For this review, take the finished solid that the model builds, in its own axes (mm). A direction names the side the tool comes from. Coordinates: 2 decimals unless noted, no trailing zeros. Order: outer loops, then holes, each group sorted by start corner. A loop starts at its lowest first (then second) coordinate and runs counter-clockwise, first axis right, second up. Notation, with made-up numbers: (67, 77) -> (93, 77) arc R20 cw to (93, 106) -> close; hole circle Ø6 at (59, 30.25). An arc over 180 degrees is marked (long way). Return JSON: item names as keys, results as strings. Group by question number.
Item 1: Take a section at B-B (z = -8.3). Write out the cut boundary in (x, y), then the cut area to 3 significant figures.
Item 2: Machinability: for faces 4 (the flat face through (11.1, 15, 2.4)), 5 (the cylindrical face through (21.2, 1.48, 11.65)), 6 (the cylindrical face through (-22, 3.04, -21.87)), 7 (the flat face through (-13.5, 11, -4)), 8 (the flat face through (0, 0, 0)), which of the approach directions +Z, -Z, +X, -X, +Y, -Y give a long, thin tool a straight path to every point of the face, cutting with its end or side? Answer none if there is none.
Item 3: For line 1 along Z through (x, y) = (18.5, 4.65); line 2 along X through (y, z) = (1.55, -17.3); line 3 along Z through (x, y) = (3, 2.35), list the stretches that pass through material, from the lowest coordinate up.
Item 4: Take a section at D-D (y = 12.5). Write out the cut boundary in (x, z).
Item 5: Draft analysis for pull direction X (two halves, no side actions). For faces 1 (the flat face through (0, 8, -23.3)), 2 (the cylindrical face through (20.696, 4.521, -16.812)), 3 (the cylindrical face through (-22, 3.04, 13.27)), state which applies: +X half, -X half, draft (parallel to the pull), parting line (faces both ways), or undercut.
Item 6: Take a section at C-C (x = 5.5). Write out the cut boundary in (y, z), then the cut area to 3 significant figures.
Item 7: Take a section at A-A (x = 0). Write out the cut boundary in (y, z).
Item 8: Insertion check: pin 1 (7.5 mm diameter, centred on x = 2.5, z = -2.5, fed in from +Y); pin 2 (3.5 mm diameter, centred on y = 12.5, z = 2, fed in from -X); pin 3 (5 mm diameter, centred on x = -18.5, z = 8.7, fed in from -Y). Each pin has a flat end and moves straight along its axis. Give the tip position at first contact, or say it passes through.
```python
from build123d import *

# Parameters (mm, degrees)
SKETCH_1_W          = 27
SKETCH_1_H          = 38
SKETCH_1_R          = 7.5
SKETCH_1_R_2        = 3.5
SKETCH_1_R_3        = 1.5
EXTRUDE_1_DEPTH     = 3
SKETCH_4_W          = 10
SKETCH_4_H          = 6
EXTRUDE_3_DEPTH     = 38
SKETCH_6_R          = 2.5
CUT_EXTRUDE_3_DEPTH = 1
EXTRUDE_4_OUTLINE_W = 27
EXTRUDE_4_OUTLINE_H = 38
EXTRUDE_4_DEPTH     = 14
SKETCH_13_R         = 2.25
CUT_EXTRUDE_6_DEPTH = 10
CUT_EXTRUDE_8_DEPTH = 2
FILLET_1_R          = 5
SKETCH_17_R         = 4
CUT_EXTRUDE_9_DEPTH = 3


# Read off the part's stored shape, not the designer's step: 凸台-拉伸4
with BuildPart() as part:
    # 草图1 → 凸台-拉伸1 (new body)
    with BuildSketch(Plane(origin=(0, 0, 0), x_dir=(1, 0, 0), z_dir=(0, 1, 0))):
        with Locations((0, 4.3)):
            Rectangle(SKETCH_1_W, SKETCH_1_H)
        with Locations(Location((0, 8.3, 0), (0, 0, 270))):
            Circle(SKETCH_1_R, mode=Mode.SUBTRACT)
        with Locations(Location((0, -5.5, 0), (0, 0, 270))):
            Circle(SKETCH_1_R_2, mode=Mode.SUBTRACT)
        with Locations(Location((-9.5, 0, 0), (0, 0, 90))):
            Circle(SKETCH_1_R_3, mode=Mode.SUBTRACT)
        with Locations(Location((-3, -10, 0), (0, 0, 90))):
            Circle(SKETCH_1_R_3, mode=Mode.SUBTRACT)
        with Locations(Location((9.5, 0, 0), (0, 0, 270))):
            Circle(SKETCH_1_R_3, mode=Mode.SUBTRACT)
        with Locations(Location((3, -10, 0), (0, 0, 270))):
            Circle(SKETCH_1_R_3, mode=Mode.SUBTRACT)
    extrude(amount=EXTRUDE_1_DEPTH)

    # 草图4 → 凸台-拉伸3 (add)
    with BuildSketch(Plane(origin=(0, 0, -23.3), x_dir=(-1, 0, 0), z_dir=(0, 0, -1))):
        with Locations((-18.5, 3)):
            Rectangle(SKETCH_4_W, SKETCH_4_H)
        with Locations((18.5, 3)):
            Rectangle(SKETCH_4_W, SKETCH_4_H)
    extrude(amount=-EXTRUDE_3_DEPTH)

    # 草图6 → 切除-拉伸3 (cut)
    with BuildSketch(Plane.XZ):
        with Locations(Location((-9.5, 0, 0), (0, 0, 270))):
            Circle(SKETCH_6_R)
        with Locations(Location((9.5, 0, 0), (0, 0, 270))):
            Circle(SKETCH_6_R)
    extrude(amount=-CUT_EXTRUDE_3_DEPTH, mode=Mode.SUBTRACT)

    # 凸台-拉伸4 outline → 凸台-拉伸4 (add)
    with BuildSketch(Plane(origin=(0, 3, 0), x_dir=(1, 0, 0), z_dir=(0, 1, 0))):
        with Locations((0, 4.3)):
            Rectangle(EXTRUDE_4_OUTLINE_W, EXTRUDE_4_OUTLINE_H)
        with BuildLine():
            ThreePointArc((-1.503424688, -10.10130318), (-3.38489666, -11.449777418), (-4.349746722, -9.345642463))
            ThreePointArc((-4.349746722, -9.345642463), (-10.420144831, -3.565242203), (-10.95445115, 4.8))
            ThreePointArc((-10.95445115, 4.8), (0, 19.8), (10.95445115, 4.8))
            ThreePointArc((10.95445115, 4.8), (10.420144831, -3.565242203), (4.349746722, -9.345642463))
            ThreePointArc((4.349746722, -9.345642463), (3.38489666, -11.449777418), (1.503424688, -10.10130318))
            ThreePointArc((1.503424688, -10.10130318), (0, -10.2), (-1.503424688, -10.10130318))
        make_face(mode=Mode.SUBTRACT)
    extrude(amount=EXTRUDE_4_DEPTH)

    # 草图13 → 切除-拉伸6 (cut)
    with BuildSketch(Plane(origin=(0, 6, 0), x_dir=(1, 0, 0), z_dir=(0, 1, 0))):
        with Locations(Location((-18.5, 17.3, 0), (0, 0, 180))):
            Circle(SKETCH_13_R)
        with Locations(Location((-18.5, -8.7, 0), (0, 0, 180))):
            Circle(SKETCH_13_R)
        with Locations(Location((18.5, -8.7, 0), (0, 0, 90))):
            Circle(SKETCH_13_R)
        with Locations(Location((18.5, 17.3, 0), (0, 0, 90))):
            Circle(SKETCH_13_R)
    extrude(amount=-CUT_EXTRUDE_6_DEPTH, mode=Mode.SUBTRACT)

    # 草图15 → 切除-拉伸8 (cut)
    with BuildSketch(Plane(origin=(0, 17, 0), x_dir=(1, 0, 0), z_dir=(0, 1, 0))):
        with BuildLine():
            ThreePointArc((11.66190379, 3.8), (0, 20.8), (-11.66190379, 3.8))
            ThreePointArc((-11.66190379, 3.8), (0, -13.2), (11.66190379, 3.8))
        make_face()
    extrude(amount=-CUT_EXTRUDE_8_DEPTH, mode=Mode.SUBTRACT)

    # 圆角1
    fillet_1_edges = [part.edges().sort_by_distance(p)[0] for p in [
        (23.5, 3, -23.3),
        (23.5, 3, 14.7),
        (-23.5, 3, -23.3),
        (-23.5, 3, 14.7),
    ]]
    fillet(fillet_1_edges, radius=FILLET_1_R)

    # 草图17 → 切除-拉伸9 (cut)
    with BuildSketch(Plane.XZ):
        with Locations(Location((-18.5, 8.7, 0), (0, 0, 270))):
            Circle(SKETCH_17_R)
        with Locations(Location((18.5, 8.7, 0), (0, 0, 270))):
            Circle(SKETCH_17_R)
        with Locations(Location((18.5, -17.3, 0), (0, 0, 270))):
            Circle(SKETCH_17_R)
        with Locations(Location((-18.5, -17.3, 0), (0, 0, 270))):
            Circle(SKETCH_17_R)
    extrude(amount=-CUT_EXTRUDE_9_DEPTH, mode=Mode.SUBTRACT)


solid = part.part
```
Findings below:
{
 "1": {"outline": "(-23.5, 0) -> (-7.5, 0) -> (-7.5, 3) -> (-11.5, 3) -> (-11.5, 15) -> (-12.5, 15) -> (-12.5, 17) -> (-13.5, 17) -> (-13.5, 6) -> (-23.5, 6) -> close; (7.5, 0) -> (23.5, 0) -> (23.5, 6) -> (13.5, 6) -> (13.5, 17) -> (12.5, 17) -> (12.5, 15) -> (11.5, 15) -> (11.5, 3) -> (7.5, 3) -> close", "area": "208 mm2"},
 "2": {"face 4": "+Y", "face 5": "-Y", "face 6": "-Z, -X, +Y, -Y", "face 7": "+Z, -Z, -X, +Y", "face 8": "+Z, -Z, +X, -X, -Y"},
 "3": {"line 1": "z = -23.3 to -19.55, -15.05 to 6.45, 10.95 to 14.7", "line 2": "x = -23.5 to -22.5, -14.5 to 14.5, 22.5 to 23.5", "line 3": "z = -23.3 to -15.17, -1.43 to 3.7, 7.3 to 8.5, 11.5 to 14.7"},
 "4": {"outline": "(-13.5, -23.3) -> (13.5, -23.3) -> (13.5, 14.7) -> (-13.5, 14.7) -> close; hole (-10.95, -4.8) arc R11.5 ccw (long way) to (10.95, -4.8) arc R11.5 ccw to (4.35, 9.35) arc R1.5 ccw (long way) to (1.5, 10.1) arc R11.5 ccw to (-1.5, 10.1) arc R1.5 ccw (long way) to (-4.35, 9.35) arc R11.5 ccw to start"},
 "5": {"face 1": "draft", "face 2": "undercut", "face 3": "-X half"},
 "6": {"outline": "(0, -23.3) -> (17, -23.3) -> (17, -19.52) -> (15, -19.52) -> (15, -18.4) -> (3, -18.4) -> (3, -13.4) -> (0, -13.4) -> close; (0, -3.2) -> (3, -3.2) -> (3, 8.8) -> (15, 8.8) -> (15, 11.92) -> (17, 11.92) -> (17, 14.7) -> (0, 14.7) -> close", "area": "226 mm2"},
 "7": {"outline": "(0, -23.3) -> (17, -23.3) -> (17, -20.8) -> (15, -20.8) -> (15, -19.8) -> (3, -19.8) -> (3, -15.8) -> (0, -15.8) -> close; (0, -0.8) -> (3, -0.8) -> (3, 2) -> (0, 2) -> close; (0, 9) -> (3, 9) -> (3, 10.2) -> (15, 10.2) -> (15, 13.2) -> (17, 13.2) -> (17, 14.7) -> (0, 14.7) -> close"},
 "8": {"pin 1": "stops at y = 3", "pin 2": "stops at x = -13.5", "pin 3": "stops at y = 3"}
}
